Check sheet for the modelled part. Datum: model origin and axes. Units: mm. A direction names the side the tool comes from. Round coordinates to 2 decimals unless told otherwise and drop trailing zeros. Write each loop counter-clockwise with the first axis right and the second up, starting at its lowest first coordinate (ties: lowest second). Pieces come first, ordered by that corner, then holes. Notation, with made-up numbers: (-2.75, -11.5) -> (44.25, -11.5) arc R31 cw to (44.25, 15.5) -> close; hole circle Ø9 at (74.25, 10). An arc over 180 degrees is marked (long way). Answer as a JSON object with one key per item and string values. Group by question number.
```python
from build123d import *

# Parameters (mm, degrees)
SKETCH1_R           = 3.25
SKETCH1_R_2         = 2.75
BOSS_EXTRUDE1_DEPTH = 3


with BuildPart() as part:
    # Sketch1 → Boss-Extrude1 (new body)
    with BuildSketch(Plane(origin=(0, 0, 0), x_dir=(1, 0, 0), z_dir=(0, 1, 0))):
        Polygon((-32.478065847, 0), (-32.478065847, 10), (-2.478065847, 10), (-2.478065847, 15), (27.521934153, 15), (27.521934153, 10), (57.521934153, 10), (57.521934153, 0), (27.521934153, 0), (27.521934153, -5), (-2.478065847, -5), (-2.478065847, 0), align=None)
        with Locations((-19.778065847, 5)):
            Circle(SKETCH1_R, mode=Mode.SUBTRACT)
        with Locations((44.821934153, 5)):
            Circle(SKETCH1_R_2, mode=Mode.SUBTRACT)
    extrude(amount=BOSS_EXTRUDE1_DEPTH)


solid = part.part
```
(1) Go/stop test with flat-tipped pins: pin 1 Ø12 at (x, z) = (-19.5, 0) entering from -Y; pin 2 Ø1.5 at (y, z) = (1, 3.5) entering from +X; pin 3 Ø1.5 at (x, y) = (35.5, 2) entering from -Z; pin 4 Ø1.5 at (x, y) = (45, 2) entering from +Z. Record where each tip stops, or that it passes through.
(2) Section check A-A on z = -5. Record the cut outline in (x, y), then the cut area to 3 significant figures.
(3) Scan lines: line 1 along X through (y, z) = (0.85, -5); line 2 along X through (y, z) = (1.75, -2.5); line 3 along Z through (x, y) = (40.5, 0.85). Record each from-to range of solid material in increasing order.
(4) Section check B-B on y = 2. Record the cut outline in (x, z), then the cut area to 3 significant figures.
(5) Section check C-C on x = 38.5. Record the cut outline in (y, z).
(6) Release check for a two-part mould opening along Z. For faces 1 (the flat face through (-2.478, 1, -12)), 2 (the cylindrical face through (47.362, 1.479, -3.947)), 3 (the flat face through (42, 1, -10)) record: pulls with the +Z half, pulls with the -Z half, needs draft (parallel to the pull), parting line crosses it, or undercut.
(7) Section check D-D on z = 1.5. Record the cut outline in (x, y), then the cut area to 3 significant figures.
(8) Access from +Z, -Z, +X, -X, +Y, -Y to the whole of each face (thin tool, end or side, straight path). Record for faces 4 (the flat face through (-2.478, 1, 3)), 5 (the flat face through (-18, 1, -10)), 6 (the flat face through (27.522, 1, -13)), 7 (the flat face through (27.522, 1, 2)).
Data:
{
 "1": {"pin 1": "stops at y = 0", "pin 2": "stops at x = 27.52", "pin 3": "stops at z = -10", "pin 4": "stops at z = 0"},
 "2": {"outline": "(-32.48, 0) -> (-23.03, 0) -> (-23.03, 3) -> (-32.48, 3) -> close; (-16.53, 0) -> (42.07, 0) -> (42.07, 3) -> (-16.53, 3) -> close; (47.57, 0) -> (57.52, 0) -> (57.52, 3) -> (47.57, 3) -> close", "area": "234 mm²"},
 "3": {"line 1": "x = -32.48 to -23.03, -16.53 to 42.07, 47.57 to 57.52", "line 2": "x = -32.48 to -21.85, -17.7 to 43.68, 45.97 to 57.52", "line 3": "z = -10 to 0"},
 "4": {"outline": "(-32.48, -10) -> (-2.48, -10) -> (-2.48, -15) -> (27.52, -15) -> (27.52, -10) -> (57.52, -10) -> (57.52, 0) -> (27.52, 0) -> (27.52, 5) -> (-2.48, 5) -> (-2.48, 0) -> (-32.48, 0) -> close; hole circle Ø6.5 at (-19.78, -5); hole circle Ø5.5 at (44.82, -5)", "area": "1,140 mm²"},
 "5": {"outline": "(0, -10) -> (3, -10) -> (3, 0) -> (0, 0) -> close"},
 "6": {"face 1": "needs draft", "face 2": "undercut", "face 3": "pulls with the -Z half"},
 "7": {"outline": "(-2.48, 0) -> (27.52, 0) -> (27.52, 3) -> (-2.48, 3) -> close", "area": "90.0 mm²"},
 "8": {"face 4": "+Z, -X, +Y, -Y", "face 5": "-Z, -X, +Y, -Y", "face 6": "-Z, +X, +Y, -Y", "face 7": "+Z, +X, +Y, -Y"}
}
